```python
from build123d import *

# Parameters (mm, degrees)
BOSS_EXTRUDE1_DEPTH = 79
SKETCH2_R           = 1.4
CUT_EXTRUDE1_DEPTH  = 79


with BuildPart() as part:
    # Sketch1 → Boss-Extrude1 (new body)
    with BuildSketch(Plane.XY):
        Polygon((-4, 10), (-6, 10), (-6, -15), (-4, -15), (-4, -10), (4, -10), (4, 10), align=None)
    extrude(amount=BOSS_EXTRUDE1_DEPTH)

    # Sketch2 → Cut-Extrude1 (cut)
    with BuildSketch(Plane(origin=(0, 0, 0), x_dir=(-1, 0, 0), z_dir=(0, 0, -1))):
        with Locations((0, 6)):
            Circle(SKETCH2_R)
        with Locations((0, -6)):
            Circle(SKETCH2_R)
    extrude(amount=-CUT_EXTRUDE1_DEPTH, mode=Mode.SUBTRACT)


solid = part.part
```
Part model, mm, in its own coordinate system. A direction names the side the tool comes from. Round coordinates to 2 decimals unless told otherwise and drop trailing zeros. Write each loop counter-clockwise with the first axis right and the second up, starting at its lowest first coordinate (ties: lowest second). Pieces come first, ordered by that corner, then holes.
Item 1: Cut at A-A, the plane x = 0. Give the cut face in (y, z).
Results:
outline: (-10, 0) - (-7.4, 0) - (-7.4, 79) - (-10, 79) - close; (-4.6, 0) - (4.6, 0) - (4.6, 79) - (-4.6, 79) - close; (7.4, 0) - (10, 0) - (10, 79) - (7.4, 79) - close
Item 2: Probe L1, parallel to Y at x = 0, z = 38; L2, parallel to Y at x = -1.75, z = 20; L3, parallel to Y at x = -0.5, z = 26.5. List the from-to ranges inside material, lowest first.
Results:
L1: y = -10 to -7.4, -4.6 to 4.6, 7.4 to 10
L2: y = -10 to 10
L3: y = -10 to -7.31, -4.69 to 4.69, 7.31 to 10
Item 3: Cut at C-C, the plane z = 21.5. Give the cut face in (x, y).
Results:
outline: (-6, -15) - (-4, -15) - (-4, -10) - (4, -10) - (4, 10) - (-6, 10) - close; hole circle Ø2.8 at (0, -6); hole circle Ø2.8 at (0, 6)
Item 4: Cut at B-B, the plane y = 6. Give the cut face in (x, z).
Results:
outline: (-6, 0) - (-1.4, 0) - (-1.4, 79) - (-6, 79) - close; (1.4, 0) - (4, 0) - (4, 79) - (1.4, 79) - close
Item 5: Cut at D-D, the plane x = -3.25. Give the cut face in (y, z).
Results:
outline: (-10, 0) - (10, 0) - (10, 79) - (-10, 79) - close
Item 6: Drop flat-ended pins along their axis: pin 1 Ø1 at (x, z) = (-3, 12.5) entering from -Y; pin 2 Ø3.5 at (x, y) = (0, 6) entering from +Z; pin 3 Ø2.5 at (y, z) = (-13, 55.5) entering from +X; pin 4 Ø2 at (x, y) = (0, -6) entering from -Z. Give the stop position or say it passes through.
Results:
pin 1: stops at y = -10
pin 2: stops at z = 79
pin 3: stops at x = -4
pin 4: passes through
Item 7: Two-plate mould, pull along Y, no slides. Class faces 3 (the flat face through (-1, 0, 0)), 4 (the flat face through (-1, 10, 39)), 5 (the cylindrical face through (0.303, -7.367, 38.947)), 6 (the flat face through (0, -10, 39)): +Y half, -Y half, draft (parallel to the pull), parting line (faces both ways), or undercut.
Results:
face 3: draft
face 4: +Y half
face 5: undercut
face 6: -Y half
Item 8: Which spindle directions (+Z, -Z, +X, -X, +Y, -Y) get a long thin tool onto all of the face, cutting with end or side? Do faces 1 (the flat face through (-4, -13, 39)), 2 (the flat face through (-6, -2, 39)). Say none if no direction does.
Results:
face 1: +Z, -Z, +X, -Y
face 2: +Z, -Z, -X, +Y, -Y
